Design review of the part shown in the three views and the two pictorial views. Dimensions are in mm from the part's minimum x, y and z. Give positions to 0.01 mm unless a question says otherwise; leave off trailing zeros. Loops run counter-clockwise (first coordinate to the right, second up) from the corner with the lowest first, then second, coordinate; pieces in that order, holes last.
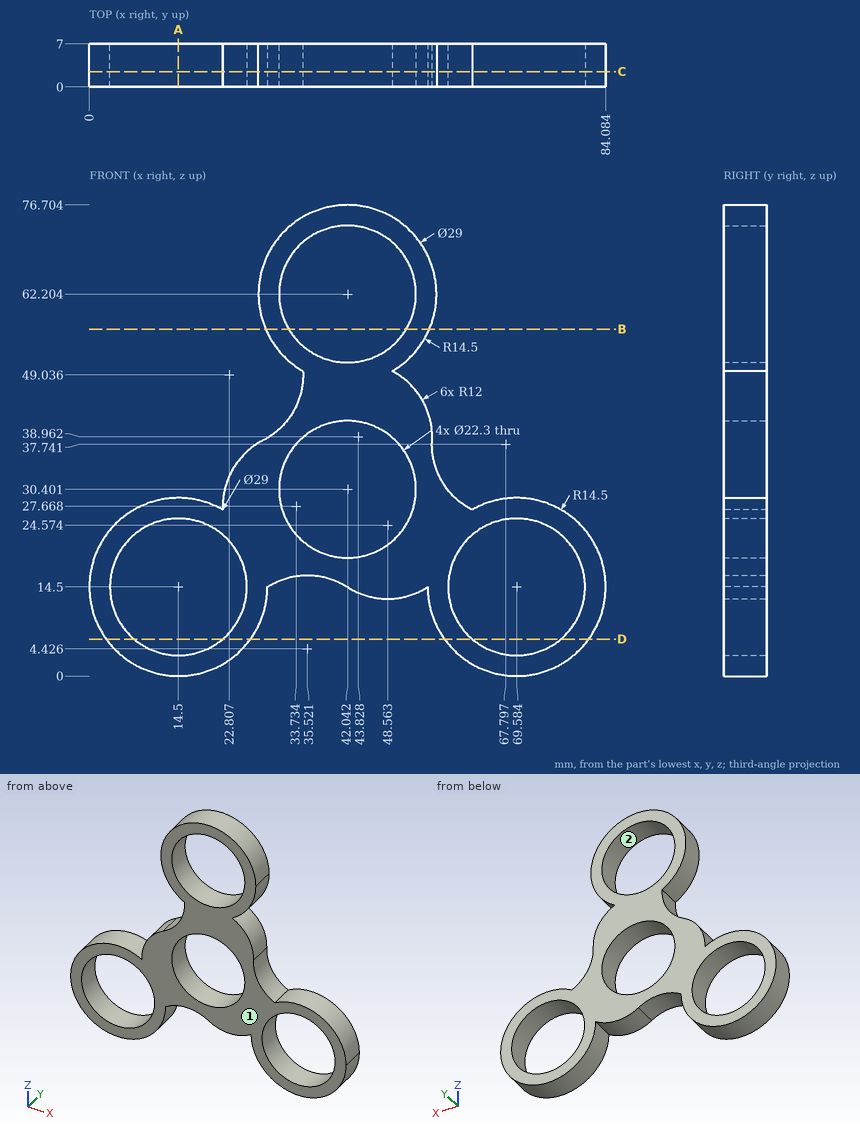
Q1. Take a section at A-A (x = 14.5). Give the boundary of the cut face in (y, z), plus the area to 3 significant figures.
Results:
outline: (0, 0) - (7, 0) - (7, 3.35) - (0, 3.35) - close; (0, 25.65) - (7, 25.65) - (7, 29) - (0, 29) - close
area: 46.9 mm2
Q2. Wall thickness on line 1 (X direction, y = 2.5, z = 10.5) (1 decimal); line 2 (Z direction, x = 40, y = 5.5) (1 decimal); line 3 (X direction, y = 5, z = 62): over which ranges is each line inside the solid? List them lowest first.
Results:
line 1: x = 0.6 to 4.1, 24.9 to 28.4, 55.6 to 59.2, 80 to 83.5
line 2: z = 15.6 to 19.4, 41.4 to 51.2, 73.2 to 76.6
line 3: x = 27.54 to 30.89, 53.19 to 56.54
Q3. Take a section at C-C (y = 2.5). Give the number of separate pieces and of enclosed holes in the cut face, plus the area to 3 significant figures.
Results:
separate pieces: 1
enclosed holes: 4
area: 1,400 mm2
Q4. Take a section at B-B (z = 56.5). Give the boundary of the cut face in (x, y).
Results:
outline: (28.71, 0) - (32.46, 0) - (32.46, 7) - (28.71, 7) - close; (51.62, 0) - (55.37, 0) - (55.37, 7) - (51.62, 7) - close
Q5. Take a section at D-D (z = 6). Give the boundary of the cut face in (x, y), plus the area to 3 significant figures.
Results:
outline: (2.75, 0) - (7.28, 0) - (7.28, 7) - (2.75, 7) - close; (21.72, 0) - (26.25, 0) - (26.25, 7) - (21.72, 7) - close; (57.84, 0) - (62.37, 0) - (62.37, 7) - (57.84, 7) - close; (76.8, 0) - (81.33, 0) - (81.33, 7) - (76.8, 7) - close
area: 127 mm2
Q6. Insertion check: pin 1 (1 mm diameter, centred on x = 36, y = 5, fed in from -Z); pin 2 (2 mm diameter, centred on y = 3, z = 54.5, fed in from -X) (1 decimal); pin 3 (1.5 mm diameter, centred on x = 56.5, y = 2, fed in from -Z) (1 decimal); pin 4 (18 mm diameter, centred on x = 14.5, z = 14.5, fed in from +Y). Each pin has a flat end and moves straight along its axis. Give the tip position at first contact, or say it passes through.
Results:
pin 1: stops at z = 16.39
pin 2: stops at x = 29.2
pin 3: stops at z = 6.9
pin 4: passes through
Q7. Draft analysis for pull direction X (two halves, no side actions). For the marked faces 1 and 2, state which applies: pulls with the +X half, pulls with the -X half, needs draft (parallel to the pull), parting line crosses it, or undercut.
Results:
face 1: needs draft
face 2: undercut
